from build123d import *

# Parameters (mm, degrees)
SKETCH_6_W          = 94.5
SKETCH_6_H          = 55
EXTRUDE_1_DEPTH     = 2
SKETCH_772_W        = 40
SKETCH_772_H        = 6
SKETCH_772_W_2      = 48
CUT_EXTRUDE_1_DEPTH = 75.571373034
JOY_R               = 1.6
CUT_EXTRUDE_2_DEPTH = 75.571373034
NANO_R              = 0.75
CUT_EXTRUDE_4_DEPTH = 75.571373034
SKETCH_648_R        = 0.75
CUT_EXTRUDE_5_DEPTH = 75.571373034
SKETCH_7_W          = 7
SKETCH_7_H          = 17
SKETCH_7_W_2        = 4
SKETCH_7_H_2        = 22
CUT_EXTRUDE_6_DEPTH = 75.571373034
CUT_EXTRUDE_7_DEPTH = 75.571373034
SKETCH_10_W         = 90.5
SKETCH_10_H         = 1
SKETCH_10_W_2       = 80.5
CUT_EXTRUDE_8_DEPTH = 75.571373175
FILLET_3_R          = 1
FILLET_START        = -1
FILLET_4_DEPTH      = 4
FILLET_4_2_DEPTH    = 2
FILLET_5_R          = 2
FILLET_6_R          = 2.5
SKETCH_11_W         = 3
SKETCH_11_H         = 14
CUT_EXTRUDE_9_DEPTH = 75.027756944
FILLET_7_R          = 1.5
FILLET_8_R          = 4


with BuildPart() as part:
    # 草图6 → 凸台-拉伸1 (new body)
    with BuildSketch(Plane.XY):
        with Locations((15.078651685, 13.390449438)):
            Rectangle(SKETCH_6_W, SKETCH_6_H)
    extrude(amount=EXTRUDE_1_DEPTH)

    # Sketch 772 → 切除-拉伸1 (cut, through all)
    with BuildSketch(Plane.XY):
        with Locations((25.828651685, -11.109550562)):
            Rectangle(SKETCH_772_W, SKETCH_772_H)
        with Locations((31.328651685, 37.890449438)):
            Rectangle(SKETCH_772_W_2, SKETCH_772_H)
    extrude(amount=CUT_EXTRUDE_1_DEPTH, mode=Mode.SUBTRACT)

    # Joy → 切除-拉伸2 (cut, through all)
    with BuildSketch(Plane.XY):
        with Locations((-25.171348315, 22.890449438)):
            Circle(JOY_R)
        with Locations((59.328651685, 37.390449438)):
            Circle(JOY_R)
        with Locations((-25.171348315, -5.109550562)):
            Circle(JOY_R)
    extrude(amount=CUT_EXTRUDE_2_DEPTH, mode=Mode.SUBTRACT)

    # Nano → 切除-拉伸4 (cut, through all)
    with BuildSketch(Plane.XY):
        with Locations((-30.171348315, 16.390449438)):
            Circle(NANO_R)
        with Locations((9.828651685, 1.390449438)):
            Circle(NANO_R)
        with Locations((-30.171348315, 1.390449438)):
            Circle(NANO_R)
        with Locations((9.828651685, 16.390449438)):
            Circle(NANO_R)
    extrude(amount=CUT_EXTRUDE_4_DEPTH, mode=Mode.SUBTRACT)

    # Sketch 648 → 切除-拉伸5 (cut, through all)
    with BuildSketch(Plane.XY):
        with Locations((39.328651685, 12.390449438)):
            Circle(SKETCH_648_R)
        with Locations((39.328651685, 27.390449438)):
            Circle(SKETCH_648_R)
    extrude(amount=CUT_EXTRUDE_5_DEPTH, mode=Mode.SUBTRACT)

    # 草图7 → 切除-拉伸6 (cut, through all)
    with BuildSketch(Plane.XY.offset(2)):
        with Locations((58.828651685, -5.609550562)):
            Rectangle(SKETCH_7_W, SKETCH_7_H)
        Polygon((-32.171348315, -14.109550562), (-25.171348315, -14.109550562), (-25.171348315, -9.109550562), (-28.171348315, -9.109550562), (-28.171348315, -1.109550562), (-32.171348315, -1.109550562), (-32.171348315, -10.609550562), align=None)
        with Locations((-30.171348315, 29.890449438)):
            Rectangle(SKETCH_7_W_2, SKETCH_7_H_2)
    extrude(amount=-CUT_EXTRUDE_6_DEPTH, mode=Mode.SUBTRACT)

    # 草图9 → 切除-拉伸7 (cut, through all)
    with BuildSketch(Plane.XY.offset(2)):
        with BuildLine():
            Line((16.358384135, 5.546605741), (19.354312374, 8.252448685))
            Line((19.354312374, 8.252448685), (17.671340733, 8.252448685))
            Line((17.671340733, 8.252448685), (15.319954825, 5.97825988))
            add(Edge.make_bspline(
                [(15.319954825, 5.97825988), (15.209662045, 5.864263234), (14.985948929, 5.633037354), (14.771319897, 5.3933541), (14.662505102, 5.271837061)],
                knots=[0, 0, 0, 0, 0.986019789, 2, 2, 2, 2], degree=3))
            Line((14.662505102, 5.271837061), (14.627668618, 5.272671384))
            Line((14.627668618, 5.272671384), (14.627668618, 8.252448685))
            Line((14.627668618, 8.252448685), (13.255032174, 8.252448685))
            Line((13.255032174, 8.252448685), (13.255032174, 1.902448685))
            Line((13.255032174, 1.902448685), (14.627668618, 1.902448685))
            Line((14.627668618, 1.902448685), (14.627668618, 4.235041243))
            Line((14.627668618, 4.235041243), (15.391570639, 4.899124533))
            Line((15.391570639, 4.899124533), (17.921996084, 1.902448685))
            Line((17.921996084, 1.902448685), (19.53335191, 1.902448685))
            Line((19.53335191, 1.902448685), (16.358384135, 5.546605741))
        make_face()
        with BuildLine():
            Line((30.672569626, 8.252448685), (29.58639644, 6.600837965))
            add(Edge.make_bspline(
                [(29.58639644, 6.600837965), (29.512770867, 6.486048967), (29.368664533, 6.261374021), (29.16262961, 5.926527835), (28.970896691, 5.601336831), (28.850642197, 5.385664551), (28.791857671, 5.280236534)],
                knots=[0, 0, 0, 0, 1.061571746, 2.077799947, 3.060362604, 4, 4, 4, 4], degree=3))
            Line((28.791857671, 5.280236534), (28.76821775, 5.280972425))
            add(Edge.make_bspline(
                [(28.76821775, 5.280972425), (28.708109277, 5.390783537), (28.58821426, 5.609817636), (28.392410779, 5.93256056), (28.188467145, 6.25994594), (28.046996459, 6.479545222), (27.974708994, 6.591754161)],
                knots=[0, 0, 0, 0, 0.980022492, 1.954796193, 2.954959484, 4, 4, 4, 4], degree=3))
            Line((27.974708994, 6.591754161), (26.900724886, 8.252448685))
            Line((26.900724886, 8.252448685), (25.337112937, 8.252448685))
            Line((25.337112937, 8.252448685), (28.02270598, 4.558781847))
            Line((28.02270598, 4.558781847), (28.02270598, 1.902448685))
            Line((28.02270598, 1.902448685), (29.395420935, 1.902448685))
            Line((29.395420935, 1.902448685), (29.395420935, 4.58368497))
            Line((29.395420935, 4.58368497), (32.224245607, 8.252448685))
            Line((32.224245607, 8.252448685), (30.672569626, 8.252448685))
        make_face()
    extrude(amount=-CUT_EXTRUDE_7_DEPTH, mode=Mode.SUBTRACT)

    # 草图10 → 切除-拉伸8 (cut, through all)
    with BuildSketch(Plane.XY.offset(2)):
        with Locations((17.078651685, 40.390449438)):
            Rectangle(SKETCH_10_W, SKETCH_10_H)
        with Locations((15.078651685, -13.609550562)):
            Rectangle(SKETCH_10_W_2, SKETCH_10_H)
    extrude(amount=-CUT_EXTRUDE_8_DEPTH, mode=Mode.SUBTRACT)

    # 圆角3
    fillet_3_edges = [part.edges().sort_by_distance(p)[0] for p in [
        (45.828651685, -8.109550562, 1),
        (5.828651685, -8.109550562, 1),
        (55.328651685, 34.890449438, 1),
        (7.328651685, 34.890449438, 1),
    ]]
    fillet(fillet_3_edges, radius=FILLET_3_R)

    # 圆角4: read off the stored shape, not the designer's step
    # 圆角4 outline → 圆角4 (cut)
    with BuildSketch(Plane.XY.offset(FILLET_START)):
        with BuildLine():
            ThreePointArc((-26.671348315, -9.109550562), (-27.732008486, -8.670210734), (-28.171348315, -7.609550562))
            Line((-28.171348315, -7.609550562), (-28.171348315, -9.109550562))
            Line((-28.171348315, -9.109550562), (-26.671348315, -9.109550562))
        make_face()
    extrude(amount=FILLET_4_DEPTH, mode=Mode.SUBTRACT)

    # Fillet 4 2 outline → Fillet 4 2 (add)
    with BuildSketch(Plane.XY):
        with BuildLine():
            Line((-25.171348315, -9.109550562), (-26.671348315, -9.109550562))
            ThreePointArc((-26.671348315, -9.109550562), (-25.610688143, -9.54889039), (-25.171348315, -10.609550562))
            Line((-25.171348315, -10.609550562), (-25.171348315, -9.109550562))
        make_face()
    extrude(amount=FILLET_4_2_DEPTH)

    # 圆角5
    fillet_5_edges = [part.edges().sort_by_distance(p)[0] for p in [
        (55.328651685, 2.890449438, 1),
        (55.328651685, 39.890449438, 1),
        (7.328651685, 39.890449438, 1),
        (62.328651685, 39.890449438, 1),
        (45.828651685, -13.109550562, 1),
        (5.828651685, -13.109550562, 1),
        (-25.171348315, -13.109550562, 1),
        (55.328651685, -13.109550562, 1),
        (62.328651685, 2.890449438, 1),
    ]]
    fillet(fillet_5_edges, radius=FILLET_5_R)

    # 圆角6
    fillet_6_edges = [part.edges().sort_by_distance(p)[0] for p in [
        (-32.171348315, -1.109550562, 1),
        (-32.171348315, 18.890449438, 1),
    ]]
    fillet(fillet_6_edges, radius=FILLET_6_R)

    # 草图11 → 切除-拉伸9 (cut, through all)
    with BuildSketch(Plane(origin=(0, 0, 0), x_dir=(-1, 0, 0), z_dir=(0, 0, -1))):
        with Locations((26.671348315, 32.890449438)):
            Rectangle(SKETCH_11_W, SKETCH_11_H)
    extrude(amount=-CUT_EXTRUDE_9_DEPTH, mode=Mode.SUBTRACT)

    # 圆角7
    # the kernel refuses this fillet: 1.5 mm, written as the material it adds along each edge
    with BuildSketch(Plane(origin=(-25.171348315, 25.890449438, 0), x_dir=(0, 1, 0), z_dir=(0, 0, 1))) as fillet_7_piece_1:
        with BuildLine():
            CenterArc((FILLET_7_R, FILLET_7_R), FILLET_7_R, 180, 90)
            Line((0, FILLET_7_R), (0, 0))
            Line((0, 0), (FILLET_7_R, 0))
        make_face()
    extrude(amount=2)
    # the kernel refuses this fillet: 1.5 mm, written as the material it takes off along each edge
    with BuildSketch(Plane(origin=(-28.171348315, 25.890449438, -3.75), x_dir=(1, 0, 0), z_dir=(0, 0, 1))) as fillet_7_2_piece_1:
        with BuildLine():
            CenterArc((FILLET_7_R, -FILLET_7_R), FILLET_7_R, 90, 90)
            Line((0, -FILLET_7_R), (0, 0))
            Line((0, 0), (FILLET_7_R, 0))
        make_face()
    extrude(amount=9.5, mode=Mode.SUBTRACT)

    # 圆角8
    fillet_8_edges = [part.edges().sort_by_distance(p)[0] for p in [
        (-25.171348315, 39.890449438, 1),
    ]]
    fillet(fillet_8_edges, radius=FILLET_8_R)


solid = part.part
The listing builds one solid part. Answer for the finished solid, in the listing's coordinates (mm). A direction names the side the tool comes from. Round coordinates to 2 decimals unless told otherwise and drop trailing zeros. Write each loop counter-clockwise with the first axis right and the second up, starting at its lowest first coordinate (ties: lowest second). Pieces come first, ordered by that corner, then holes. Notation, with made-up numbers: (1.25, -5.75) - (21.25, -5.75) arc R15 cw to (21.25, 1.25) - close; hole circle Ø2 at (88, -38). An arc over 180 degrees is marked (long way). Use a Markdown table: item, result. Add a question column.
1. The part is cut by section A-A (x = 42.5). Write down the section's boundary in (y, z), and give its area (3 significant figures).
2. The part is cut by section C-C (z = 1.6). Give the number of separate pieces and of enclosed holes in the cut face, and give its area (3 significant figures).
3. Consider line 1 (X direction, y = 17, z = 1.3); line 2 (Y direction, x = 14, z = 0.7); line 3 (X direction, y = 12.5, z = 1.6). Determine where each line is inside the solid, lowest interval first.
4. For a pull along X with two mould halves and no side action, classify faces 1 (the face through (-23.693, -5.722, 0.986)), 2 (the face through (61.758, 3.492, 0.986)), 3 (the face through (14, 14, 0)) as +X half, -X half, draft (parallel to the pull), parting line (faces both ways), or undercut.
5. A tool of negligible diameter and unlimited length cuts with its end or side. For faces 4 (the face through (26, -8.11, 1)), 5 (the face through (59, 2.89, 1)), 6 (the face through (55.329, 37, 1)), 7 (the face through (29.395, 3, 1)), 8 (the face through (-28.171, 22, 1)), from which of +Z, -Z, +X, -X, +Y, -Y can it reach the whole face along a straight path? Write none if from no direction.
6. Flat-ended cylindrical pins translate along their axes: P1, Ø1.2, axis at x = 32, z = 1.5, coming from the -Y side; P2, Ø0.5, axis at x = -28.5, z = 0.5, coming from the +Y side; P3, Ø2.5, axis at x = -25.17, y = -5.11, coming from the +Z side; P4, Ø1, axis at y = -7.5, z = 1, coming from the +X side. Find the tip coordinate at first contact, or state that the pin passes through.
7. The part is cut by section B-B (y = 31.5). Write down the section's boundary in (x, z), and give its area (3 significant figures).
Reported:
| question | item | result |
|---|---|---|
| 1 | outline | (-8.11, 0) - (34.89, 0) - (34.89, 2) - (-8.11, 2) - close |
| 1 | area | 86.0 mm^2 |
| 2 | separate pieces | 1 |
| 2 | enclosed holes | 11 |
| 2 | area | 4,190 mm^2 |
| 3 | line 1 | -32.1 to -30.61, -29.73 to 9.39, 10.27 to 62.33 |
| 3 | line 2 | -8.11 to 1.9, 8.25 to 34.89 |
| 3 | line 3 | -32.17 to 38.59, 40.07 to 62.33 |
| 4 | face 1 | undercut |
| 4 | face 2 | +X half |
| 4 | face 3 | draft |
| 5 | face 4 | +Z, -Z, -Y |
| 5 | face 5 | +Z, -Z, +X, -Y |
| 5 | face 6 | +Z, -Z, +Y |
| 5 | face 7 | +Z, -Z |
| 5 | face 8 | +Z, -Z, -X, +Y |
| 6 | P1 | y = -8.11 |
| 6 | P2 | y = 18.89 |
| 6 | P3 | through |
| 6 | P4 | x = 55.33 |
| 7 | outline | (-25.17, 0) - (62.33, 0) - (62.33, 2) - (-25.17, 2) - close |
| 7 | area | 175 mm^2 |
